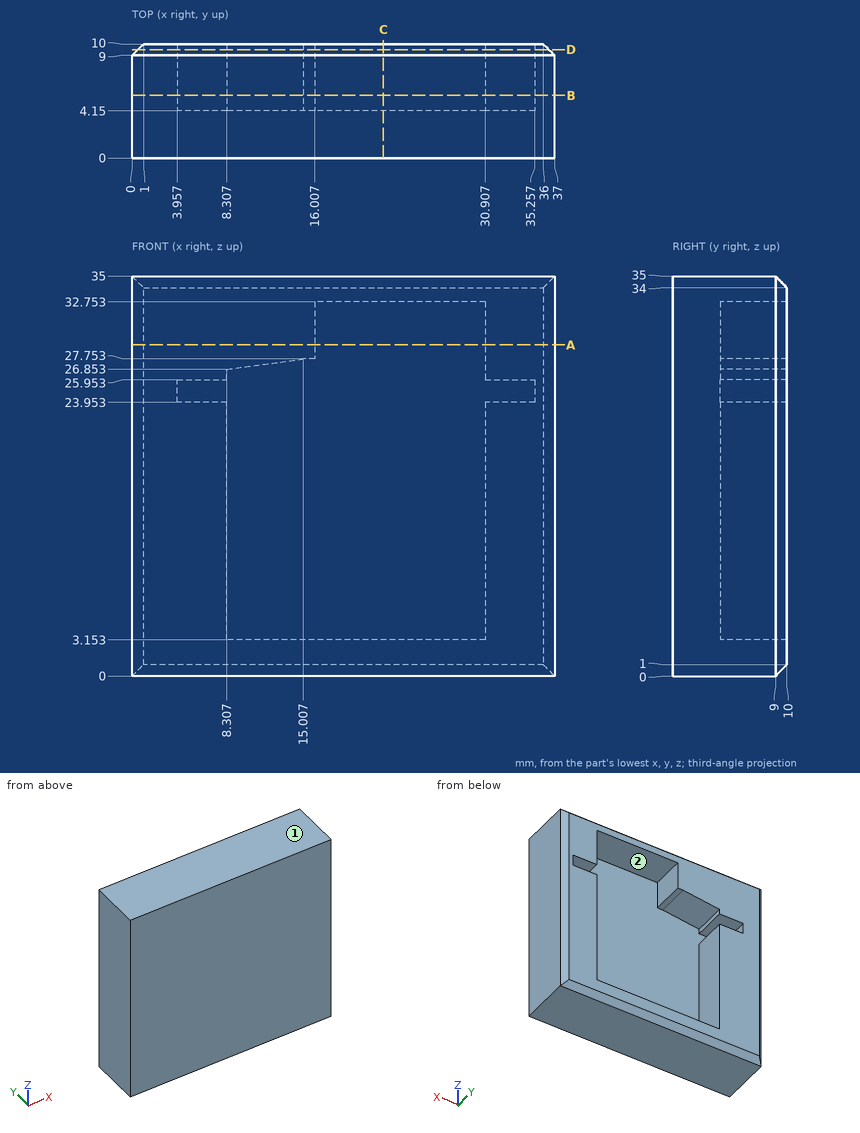
Geometry check sheet. Reference: drawing and pictorial views, mm from the part's lowest x, y, z. A direction names the side the tool comes from. Give positions to 0.01 mm unless a question says otherwise; leave off trailing zeros. Order: outer loops, then holes, each group sorted by start corner. A loop starts at its lowest first (then second) coordinate and runs counter-clockwise, first axis right, second up. Notation, with made-up numbers: M -16.5,-3 L 42.5,-3 A26 cw 42.5,20 Z; hole C -2.75,-13 d6. An arc over 180 degrees is marked long. Answer in a Markdown table with one row per item.
1) Cross-section at D-D, the plane y = 9.5. Enter the section's corners in (x, z).
Filled sheet:
| item | result |
|---|---|
| outline | M 0.5,0.5 L 36.5,0.5 L 36.5,34.5 L 0.5,34.5 Z; hole M 3.96,23.95 L 8.31,23.95 L 8.31,3.15 L 30.91,3.15 L 30.91,23.95 L 35.26,23.95 L 35.26,25.95 L 30.91,25.95 L 30.91,32.75 L 16.01,32.75 L 16.01,27.75 L 15.01,27.75 L 8.31,26.85 L 8.31,25.95 L 3.96,25.95 Z |
2) Cross-section at C-C, the plane x = 22. Enter the section's corners in (y, z), plus the area to 3 significant figures.
Filled sheet:
| item | result |
|---|---|
| outline | M 0,0 L 9,0 L 10,1 L 10,3.15 L 4.15,3.15 L 4.15,32.75 L 10,32.75 L 10,34 L 9,35 L 0,35 Z |
| area | 176 mm2 |
3) Gauge pin test, flat end, axial feed: P1, Ø1.5, axis at x = 32, z = 27.5, coming from the -Y side. Record the tip position at first contact, or that the pin passes through.
Filled sheet:
| item | result |
|---|---|
| P1 | stops at y = 0 |
4) Cross-section at B-B, the plane y = 5.5. Enter the section's corners in (x, z).
Filled sheet:
| item | result |
|---|---|
| outline | M 0,0 L 37,0 L 37,35 L 0,35 Z; hole M 3.96,23.95 L 8.31,23.95 L 8.31,3.15 L 30.91,3.15 L 30.91,23.95 L 35.26,23.95 L 35.26,25.95 L 30.91,25.95 L 30.91,32.75 L 16.01,32.75 L 16.01,27.75 L 15.01,27.75 L 8.31,26.85 L 8.31,25.95 L 3.96,25.95 Z |
5) Cross-section at A-A, the plane z = 29. Enter the section's corners in (x, y), plus the area to 3 significant figures.
Filled sheet:
| item | result |
|---|---|
| outline | M 0,0 L 37,0 L 37,9 L 36,10 L 30.91,10 L 30.91,4.15 L 16.01,4.15 L 16.01,10 L 1,10 L 0,9 Z |
| area | 282 mm2 |
6) Thickness scan on L1, parallel to Z at x = 19, y = 6.75; L2, parallel to X at y = 4.25, z = 12; L3, parallel to Z at x = 4, y = 5. Record the ranges inside material, lowest first. Write a range as [from, to].
Filled sheet:
| item | result |
|---|---|
| L1 | z = [0, 3.15], [32.75, 35] |
| L2 | x = [0, 8.31], [30.91, 37] |
| L3 | z = [0, 23.95], [25.95, 35] |
7) Access from +Z, -Z, +X, -X, +Y, -Y to the whole of each face (thin tool, end or side, straight path). Record for the marked faces 1 and 2.
Filled sheet:
| item | result |
|---|---|
| face 1 | +Z, +X, -X, +Y, -Y |
| face 2 | +Y |
